Geometry: final body of the model. Coordinates: model frame, mm. A direction names the side the tool comes from. Round coordinates to 2 decimals unless told otherwise and drop trailing zeros. Write each loop counter-clockwise with the first axis right and the second up, starting at its lowest first coordinate (ties: lowest second). Pieces come first, ordered by that corner, then holes. Notation, with made-up numbers: M -21,11.25 L 14,11.25 A16 ccw 14,23.25 Z; hole C 7.25,74.25 d8. An arc over 180 degrees is marked long. Use one line per item in the form item = value. Start each with the question number.
Item 1: Section query B-B (x = -17). Return loops of the section in (y, z).
Item 2: Pull-direction query (Y, two-part tool) for faces 6 (the flat face through (0, -25, -33)), 7 (the flat face through (0, -34.091, 0)), 8 (the flat face through (-12, -39, 48.959)); classes: pulls with the +Y half, pulls with the -Y half, needs draft (parallel to the pull), parting line crosses it, or undercut.
Item 3: Section query C-C (x = 6.5). Return loops of the section in (y, z).
Item 4: Section query A-A (y = -36.5). Return loops of the section in (x, z), and give its area (3 significant figures).
Item 5: Section query D-D (y = -28.5). Return loops of the section in (x, z) (3 decimals), and give its area (3 significant figures).
Item 6: Ray query, probe 1 along Y at (x, z) = (-11, -1); probe 2 along Y at (x, z) = (12.5, 33.5); probe 3 along Z at (x, y) = (10, -41). Return the intervals inside material, ascending.
Item 7: Reachability of faces 1 (the flat face through (14.078, -45, -33)), 2 (the flat face through (14.078, -45, 31)), 3 (the cylindrical face through (-11.11, -57.92, -27.83)), 4 (the cylindrical face through (6.007, -20.436, 18.036)), 5 (the flat face through (-21, -52, -1)) from +Z, -Z, +X, -X, +Y, -Y: full face, straight path, thin tool, end or side. Return the list, or none.
Item 8: Pin query (flat end, axial travel): pin 1 Ø21.5 at (y, z) = (-45, -37) entering from +X; pin 2 Ø1 at (x, y) = (-15.5, -21.5) entering from +Z; pin 3 Ø8 at (y, z) = (-39.5, 31.5) entering from -X. Return the tip coordinate at first contact, or that it passes through.
from build123d import *

# Parameters (mm, degrees)
SKETCH1_R           = 20
BOSS_EXTRUDE1_DEPTH = 52
SKETCH2_R           = 29
BOSS_EXTRUDE2_DEPTH = 12
BOSS_EXTRUDE3_DEPTH = 27
CUT_EXTRUDE1_DEPTH  = 93.503464219
SKETCH8_W           = 28.411423822
SKETCH8_H           = 9
CUT_EXTRUDE2_DEPTH  = 26
SKETCH9_R           = 20.095724015
CUT_EXTRUDE3_DEPTH  = 12


with BuildPart() as part:
    # Sketch1 → Boss-Extrude1 (new body)
    with BuildSketch(Plane(origin=(0, 0, 0), x_dir=(1, 0, 0), z_dir=(0, 1, 0))):
        with Locations(Location((0, 1.040702914, 0), (0, 0, 270))):
            Circle(SKETCH1_R)
    extrude(amount=-BOSS_EXTRUDE1_DEPTH)

    # Sketch2 → Boss-Extrude2 (add)
    with BuildSketch(Plane.XZ.offset(52)):
        with Locations(Location((0, -1.040702914, 0), (0, 0, 270))):
            Circle(SKETCH2_R)
    extrude(amount=BOSS_EXTRUDE2_DEPTH)

    # Sketch5 → Boss-Extrude3 (add)
    with BuildSketch(Plane(origin=(0, -52, 0), x_dir=(1, 0, 0), z_dir=(0, 1, 0))):
        with BuildLine():
            Line((14.078272234, -13.165008997), (-14.078272234, -13.165008997))
            Line((-14.078272234, -13.165008997), (-14.078272234, -48.959297086))
            Line((-14.078272234, -48.959297086), (-8.855775068, -48.959297086))
            ThreePointArc((-8.855775068, -48.959297086), (0.001248583, -41.557149408), (8.858272234, -48.959297086))
            Line((8.858272234, -48.959297086), (14.078272234, -48.959297086))
            Line((14.078272234, -48.959297086), (14.078272234, -13.165008997))
        make_face()
        with BuildLine():
            Line((-14.078272234, 51.040702914), (-14.078272234, 15.246414825))
            Line((-14.078272234, 15.246414825), (14.078272234, 15.246414825))
            Line((14.078272234, 15.246414825), (14.078272234, 51.040702914))
            Line((14.078272234, 51.040702914), (9.144224932, 51.040702914))
            ThreePointArc((9.144224932, 51.040702914), (0.144224932, 42.040702914), (-8.855775068, 51.040702914))
            Line((-8.855775068, 51.040702914), (-14.078272234, 51.040702914))
        make_face()
    extrude(amount=BOSS_EXTRUDE3_DEPTH)

    # Sketch6 → Cut-Extrude1 (cut, through all)
    with BuildSketch(Plane(origin=(14.078272234, 0, 0), x_dir=(0, 0, -1), z_dir=(1, 0, 0))):
        Polygon((-13.165008997, -34.09107024), (-37.484236428, -34.09107024), (-37.484236428, -43.09107024), (36.957800208, -43.09107024), (36.957800208, -34.09107024), align=None)
    extrude(amount=-CUT_EXTRUDE1_DEPTH, mode=Mode.SUBTRACT)

    # Sketch8 → Cut-Extrude2 (cut, symmetric)
    with BuildSketch(Plane(origin=(0, 0, 0), x_dir=(0, 0, -1), z_dir=(1, 0, 0))):
        with Locations((1.040702914, -38.59107024)):
            Rectangle(SKETCH8_W, SKETCH8_H)
    extrude(amount=CUT_EXTRUDE2_DEPTH, both=True, mode=Mode.SUBTRACT)

    # Sketch9 → Cut-Extrude3 (cut)
    with BuildSketch(Plane(origin=(0, 0, 0), x_dir=(1, 0, 0), z_dir=(0, 1, 0))):
        with Locations((0, 1.040702914)):
            Circle(SKETCH9_R)
    extrude(amount=-CUT_EXTRUDE3_DEPTH, mode=Mode.SUBTRACT)


solid = part.part
Working result:
q1.outline = M -64,-24.54 L -52,-24.54 L -52,-11.58 L -43.09,-11.58 L -43.09,9.49 L -52,9.49 L -52,22.45 L -64,22.45 Z; M -34.09,-11.58 L -12,-11.58 L -12,9.49 L -34.09,9.49 Z
q2.face_6 = pulls with the +Y half
q2.face_7 = undercut
q2.face_8 = needs draft
q3.outline = M -64,-29.3 L -52,-29.3 L -52,-44.67 L -25,-44.67 L -25,-19.95 L -12,-19.95 L -12,17.87 L -25,17.87 L -25,44.33 L -52,44.33 L -52,27.22 L -64,27.22 Z; hole M -43.09,-36.96 L -34.09,-36.96 L -34.09,37.48 L -43.09,37.48 Z
q4.outline = M -14.08,-51.04 L -8.86,-51.04 A9 cw 9.14,-51.04 L 14.08,-51.04 L 14.08,-36.96 L -14.08,-36.96 Z; M -14.08,37.48 L 14.08,37.48 L 14.08,48.96 L 8.86,48.96 A9 cw -8.86,48.96 L -14.08,48.96 Z
q4.area = 494 mm²
q5.outline = M -14.078,-51.041 L -8.856,-51.041 A9 cw 9.144,-51.041 L 14.078,-51.041 L 14.078,-15.246 A20 ccw 14.078,13.165 L 14.078,48.959 L 8.858,48.959 A9 cw -8.856,48.959 L -14.078,48.959 L -14.078,13.165 A20 ccw -14.078,-15.246 Z
q5.area = 2,820 mm²
q6.probe_1 = -64 to -43.09, -34.09 to -12
q6.probe_2 = -52 to -43.09, -34.09 to -25
q6.probe_3 = -51.04 to -36.96, 37.48 to 48.96
q7.face_1 = -Z, +X, +Y
q7.face_2 = +Z, +X, +Y
q7.face_3 = -Y
q7.face_4 = +Y
q7.face_5 = -X, +Y
q8.pin_1 = 14.08
q8.pin_2 = 12.19
q8.pin_3 = -14.08
